from build123d import *

# Parameters (mm, degrees)
SKICA2_W                 = 110
SKICA2_H                 = 160
P_IDAT_VYSUNUT_M1_DEPTH  = 5
SKICA3_W                 = 110
SKICA3_H                 = 5
P_IDAT_VYSUNUT_M2_DEPTH  = 30
P_IDAT_VYSUNUT_M3_DEPTH  = 5
P_IDAT_VYSUNUT_M4_DEPTH  = 5
SKICA6_R                 = 2.1
ODEBRAT_VYSUNUT_M1_DEPTH = 5
SKICA8_R                 = 1.3
SKICA8_R_2               = 1.35
ODEBRAT_VYSUNUT_M3_DEPTH = 5
SKICA9_R                 = 2.1
ODEBRAT_VYSUNUT_M4_DEPTH = 5
SKICA10_R                = 4
ODEBRAT_VYSUNUT_M5_DEPTH = 3
ZAOBLIT1_R               = 5
ZKOSEN_3_SIZE            = 0.5
ZKOSEN_6_SIZE            = 0.5
ODEBRAT_VYSUNUT_M6_DEPTH = 5
ZKOSEN_7_SIZE            = 0.5


with BuildPart() as part:
    # Skica2 → Přidat vysunutím1 (new body)
    with BuildSketch(Plane(origin=(0, 0, 0), x_dir=(1, 0, 0), z_dir=(0, 1, 0))):
        with Locations((55, 80)):
            Rectangle(SKICA2_W, SKICA2_H)
    extrude(amount=P_IDAT_VYSUNUT_M1_DEPTH)

    # Skica3 → Přidat vysunutím2 (add)
    with BuildSketch(Plane(origin=(0, 5, 0), x_dir=(1, 0, 0), z_dir=(0, 1, 0))):
        with Locations((55, 77.5)):
            Rectangle(SKICA3_W, SKICA3_H)
    extrude(amount=P_IDAT_VYSUNUT_M2_DEPTH)

    # Skica4 → Přidat vysunutím3 (add)
    with BuildSketch(Plane.ZY):
        Polygon((-75, 35), (-55, 5), (-75, 5), align=None)
    extrude(amount=-P_IDAT_VYSUNUT_M3_DEPTH)

    # Skica5 → Přidat vysunutím4 (add)
    with BuildSketch(Plane(origin=(110, 0, 0), x_dir=(0, 0, -1), z_dir=(1, 0, 0))):
        Polygon((75, 35), (55, 5), (75, 5), align=None)
    extrude(amount=-P_IDAT_VYSUNUT_M4_DEPTH)

    # Skica6 → Odebrat vysunutím1 (cut)
    with BuildSketch(Plane(origin=(0, 0, -80), x_dir=(-1, 0, 0), z_dir=(0, 0, -1))):
        with Locations((-100.2, 23.25)):
            Circle(SKICA6_R)
        with Locations((-9.8, 23.25)):
            Circle(SKICA6_R)
    extrude(amount=-ODEBRAT_VYSUNUT_M1_DEPTH, mode=Mode.SUBTRACT)

    # Skica8 → Odebrat vysunutím3 (cut)
    with BuildSketch(Plane(origin=(0, 5, 0), x_dir=(1, 0, 0), z_dir=(0, 1, 0))):
        with Locations(Location((29.55, 12, 0), (0, 0, 270))):
            Circle(SKICA8_R)
        with Locations(Location((30.82, 60.26, 0), (0, 0, 270))):
            Circle(SKICA8_R_2)
        with Locations(Location((81.62, 17.09, 0), (0, 0, 270))):
            Circle(SKICA8_R_2)
        with Locations(Location((81.62, 45.03, 0), (0, 0, 270))):
            Circle(SKICA8_R_2)
    extrude(amount=-ODEBRAT_VYSUNUT_M3_DEPTH, mode=Mode.SUBTRACT)

    # Skica9 → Odebrat vysunutím4 (cut)
    with BuildSketch(Plane.XZ):
        with Locations(Location((5.5, -5.5, 0), (0, 0, 270))):
            Circle(SKICA9_R)
        with Locations(Location((24.5, -5.5, 0), (0, 0, 270))):
            Circle(SKICA9_R)
        with Locations(Location((5.5, -29.5, 0), (0, 0, 270))):
            Circle(SKICA9_R)
        with Locations(Location((24.5, -29.5, 0), (0, 0, 270))):
            Circle(SKICA9_R)
        with Locations(Location((85.5, -29.5, 0), (0, 0, 270))):
            Circle(SKICA9_R)
        with Locations(Location((104.5, -29.5, 0), (0, 0, 270))):
            Circle(SKICA9_R)
        with Locations(Location((85.5, -5.5, 0), (0, 0, 270))):
            Circle(SKICA9_R)
        with Locations(Location((104.5, -5.5, 0), (0, 0, 270))):
            Circle(SKICA9_R)
        with Locations(Location((104.5, -154.5, 0), (0, 0, 270))):
            Circle(SKICA9_R)
        with Locations(Location((85.5, -154.5, 0), (0, 0, 270))):
            Circle(SKICA9_R)
        with Locations(Location((104.5, -130.5, 0), (0, 0, 270))):
            Circle(SKICA9_R)
        with Locations(Location((85.5, -130.5, 0), (0, 0, 270))):
            Circle(SKICA9_R)
        with Locations(Location((24.5, -130.5, 0), (0, 0, 270))):
            Circle(SKICA9_R)
        with Locations(Location((5.5, -130.5, 0), (0, 0, 270))):
            Circle(SKICA9_R)
        with Locations(Location((24.5, -154.5, 0), (0, 0, 270))):
            Circle(SKICA9_R)
        with Locations(Location((5.5, -154.5, 0), (0, 0, 270))):
            Circle(SKICA9_R)
    extrude(amount=-ODEBRAT_VYSUNUT_M4_DEPTH, mode=Mode.SUBTRACT)

    # Skica10 → Odebrat vysunutím5 (cut)
    with BuildSketch(Plane(origin=(0, 5, 0), x_dir=(1, 0, 0), z_dir=(0, 1, 0))):
        with Locations(Location((5.5, 154.5, 0), (0, 0, 270))):
            Circle(SKICA10_R)
        with Locations(Location((24.5, 154.5, 0), (0, 0, 270))):
            Circle(SKICA10_R)
        with Locations(Location((5.5, 130.5, 0), (0, 0, 270))):
            Circle(SKICA10_R)
        with Locations(Location((24.5, 130.5, 0), (0, 0, 270))):
            Circle(SKICA10_R)
        with Locations(Location((85.5, 130.5, 0), (0, 0, 90))):
            Circle(SKICA10_R)
        with Locations(Location((104.5, 130.5, 0), (0, 0, 90))):
            Circle(SKICA10_R)
        with Locations(Location((85.5, 154.5, 0), (0, 0, 90))):
            Circle(SKICA10_R)
        with Locations(Location((104.5, 154.5, 0), (0, 0, 90))):
            Circle(SKICA10_R)
        with Locations(Location((104.5, 5.5, 0), (0, 0, 270))):
            Circle(SKICA10_R)
        with Locations(Location((85.5, 5.5, 0), (0, 0, 270))):
            Circle(SKICA10_R)
        with Locations(Location((104.5, 29.5, 0), (0, 0, 270))):
            Circle(SKICA10_R)
        with Locations(Location((85.5, 29.5, 0), (0, 0, 270))):
            Circle(SKICA10_R)
        with Locations(Location((24.5, 29.5, 0), (0, 0, 90))):
            Circle(SKICA10_R)
        with Locations(Location((5.5, 29.5, 0), (0, 0, 90))):
            Circle(SKICA10_R)
        with Locations(Location((24.5, 5.5, 0), (0, 0, 90))):
            Circle(SKICA10_R)
        with Locations(Location((5.5, 5.5, 0), (0, 0, 90))):
            Circle(SKICA10_R)
    extrude(amount=-ODEBRAT_VYSUNUT_M5_DEPTH, mode=Mode.SUBTRACT)

    # Zaoblit1
    zaoblit1_edges = [part.edges().sort_by_distance(p)[0] for p in [
        (0, 2.5, -160),
        (110, 2.5, -160),
        (110, 2.5, 0),
        (0, 2.5, 0),
    ]]
    fillet(zaoblit1_edges, radius=ZAOBLIT1_R)

    # Zkosení3
    zkosen_3_edges = [part.edges().sort_by_distance(p)[0] for p in [
        (110, 5, -117.5),
        (110, 5, -30),
        (55, 5, 0),
        (1.464466094, 5, -1.464466094),
        (108.535533906, 5, -1.464466094),
        (55, 5, -160),
        (0, 5, -117.5),
        (1.464466094, 5, -158.535533906),
        (108.535533906, 5, -158.535533906),
        (0, 5, -30),
    ]]
    chamfer(zkosen_3_edges, length=ZKOSEN_3_SIZE)

    # Zkosení6
    zkosen_6_edges = [part.edges().sort_by_distance(p)[0] for p in [
        (102.3, 23.25, -80),
        (102.3, 23.25, -75),
        (11.9, 23.25, -80),
        (11.9, 23.25, -75),
    ]]
    chamfer(zkosen_6_edges, length=ZKOSEN_6_SIZE)

    # Skica11 → Odebrat vysunutím6 (cut)
    with BuildSketch(Plane(origin=(0, 5, 0), x_dir=(1, 0, 0), z_dir=(0, 1, 0))):
        with BuildLine():
            Line((34.5, 134.5), (75.5, 134.5))
            ThreePointArc((75.5, 134.5), (77.5, 132.5), (75.5, 130.5))
            Line((75.5, 130.5), (34.5, 130.5))
            ThreePointArc((34.5, 130.5), (32.5, 132.5), (34.5, 134.5))
        make_face()
        with BuildLine():
            Line((34.5, 126.5), (75.5, 126.5))
            ThreePointArc((75.5, 126.5), (77.5, 124.5), (75.5, 122.5))
            Line((75.5, 122.5), (34.5, 122.5))
            ThreePointArc((34.5, 122.5), (32.5, 124.5), (34.5, 126.5))
        make_face()
        with BuildLine():
            Line((34.5, 118.5), (75.5, 118.5))
            ThreePointArc((75.5, 118.5), (77.5, 116.5), (75.5, 114.5))
            Line((75.5, 114.5), (34.5, 114.5))
            ThreePointArc((34.5, 114.5), (32.5, 116.5), (34.5, 118.5))
        make_face()
        with BuildLine():
            Line((34.5, 110.5), (75.5, 110.5))
            ThreePointArc((75.5, 110.5), (77.5, 108.5), (75.5, 106.5))
            Line((75.5, 106.5), (34.5, 106.5))
            ThreePointArc((34.5, 106.5), (32.5, 108.5), (34.5, 110.5))
        make_face()
        with BuildLine():
            Line((34.5, 102.5), (75.5, 102.5))
            ThreePointArc((75.5, 102.5), (77.5, 100.5), (75.5, 98.5))
            Line((75.5, 98.5), (34.5, 98.5))
            ThreePointArc((34.5, 98.5), (32.5, 100.5), (34.5, 102.5))
        make_face()
        with BuildLine():
            Line((34.5, 94.5), (75.5, 94.5))
            ThreePointArc((75.5, 94.5), (77.5, 92.5), (75.5, 90.5))
            Line((75.5, 90.5), (34.5, 90.5))
            ThreePointArc((34.5, 90.5), (32.5, 92.5), (34.5, 94.5))
        make_face()
        with BuildLine():
            Line((34.5, 86.5), (75.5, 86.5))
            ThreePointArc((75.5, 86.5), (77.5, 84.5), (75.5, 82.5))
            Line((75.5, 82.5), (34.5, 82.5))
            ThreePointArc((34.5, 82.5), (32.5, 84.5), (34.5, 86.5))
        make_face()
    extrude(amount=-ODEBRAT_VYSUNUT_M6_DEPTH, mode=Mode.SUBTRACT)

    # Zkosení7
    zkosen_7_edges = [part.edges().sort_by_distance(p)[0] for p in [
        (30.82, 5, -61.61),
        (29.55, 5, -13.3),
        (81.62, 5, -18.44),
        (81.62, 5, -46.38),
    ]]
    chamfer(zkosen_7_edges, length=ZKOSEN_7_SIZE)


solid = part.part
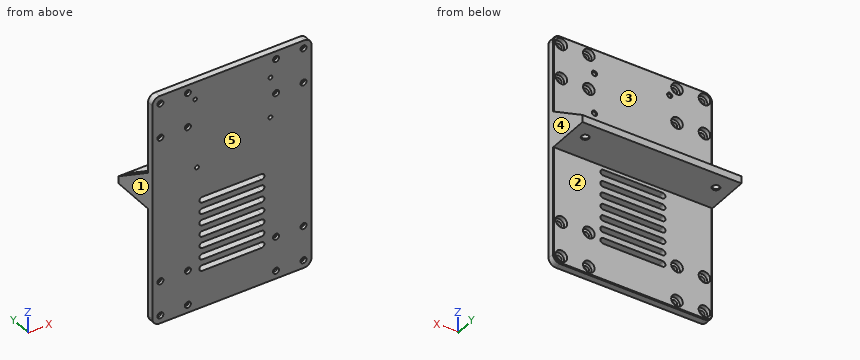
Verification items for the finished model (mm, model axes). Face numbers are marked on the shaded views. A direction names the side the tool comes from. Coordinates: 2 decimals unless noted, no trailing zeros. Write each loop counter-clockwise with the first axis right and the second up, starting at its lowest first coordinate (ties: lowest second). Pieces come first, ordered by that corner, then holes. Notation, with made-up numbers: M 42.25,86.25 L 53.25,86.25 A24 ccw 53.25,108.25 Z; hole C 78,80.25 d4. An arc over 180 degrees is marked long. One line per question, with ' | ' between items.
1) Material ranges on L1, parallel to Z at x = 81.62, y = 1.3; L2, parallel to X at y = 3.8, z = -29.5; L3, parallel to X at y = 23.5, z = -76, recorded low to high.
Solutions:
L1: -160 to -46.38, -43.68 to -18.44, -15.74 to 0 | L2: 0 to 1.5, 9.5 to 20.5, 28.5 to 81.5, 89.5 to 100.5, 108.5 to 110 | L3: 0 to 7.71, 11.89 to 98.11, 102.29 to 110
2) Depth check by flat-ended pin: pin 1 Ø6 at (x, y) = (46, 31) entering from -Z; pin 2 Ø2.5 at (x, z) = (104.5, -29.5) entering from -Y; pin 3 Ø4 at (x, z) = (7, -6.5) entering from +Y; pin 4 Ø1 at (x, y) = (21, 30.5) entering from +Z. Enter the tip coordinate at first touch or a pass-through.
Solutions:
pin 1: z = -80 | pin 2: through | pin 3: y = 2 | pin 4: z = -75
3) Sectioned sample at C-C on z = -50. Record the cut outline in (x, y), then the cut area to 3 significant figures.
Solutions:
outline: M 0,0 L 110,0 L 110,4.5 L 109.5,5 L 0.5,5 L 0,4.5 Z | area: 550 mm^2
4) Access from +Z, -Z, +X, -X, +Y, -Y to the whole of each face (thin tool, end or side, straight path). Record for the marked faces 1 and 2.
Solutions:
face 1: +Z, -Z, -X, +Y, -Y | face 2: -Z, +X, -X, +Y
5) Release check for a two-part mould opening along X. For the marked faces 3, 4 and 5 record: +X half, -X half, draft (parallel to the pull), parting line (faces both ways), or undercut.
Solutions:
face 3: undercut | face 4: +X half | face 5: draft
6) Sectioned sample at B-B on x = 85.5. State how many separate pieces and enclosed holes the cut face has, then the cut area to 3 significant figures.
Solutions:
separate pieces: 5 | enclosed holes: 0 | area: 820 mm^2
7) Sectioned sample at A-A on y = 29. Record the cut outline in (x, z), then the cut area to 3 significant figures.
Solutions:
outline: M 0,-80 L 110,-80 L 110,-71 L 105,-71 L 105,-75 L 5,-75 L 5,-71 L 0,-71 Z | area: 590 mm^2
